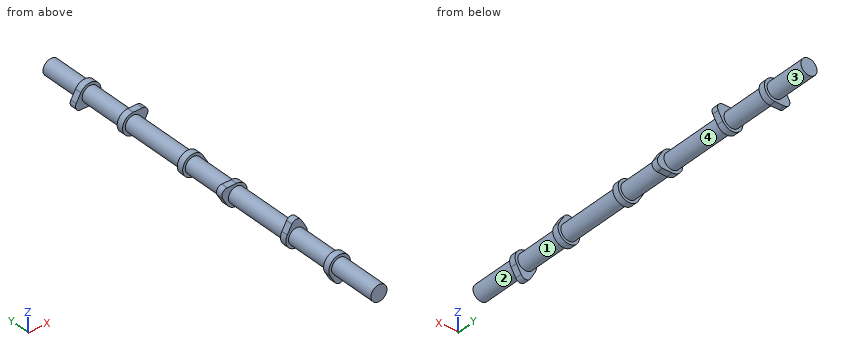
from build123d import *

# Parameters (mm, degrees)
BOSS_EXTRUDE1_DEPTH   = 3.81
LPATTERN1_COUNT       = 2
LPATTERN1_PITCH       = 60.96
BODY_MOVE_COPY1_ANGLE = 180
LPATTERN2_COUNT       = 3
LPATTERN2_PITCH       = 146.05
BODY_MOVE_COPY2_ANGLE = 120
BODY_MOVE_COPY3_ANGLE = 120
BOSS_EXTRUDE2_START   = -59.53
SKETCH5_R             = 9.5
BOSS_EXTRUDE2_DEPTH   = 464.25


with BuildPart() as part:
    # Sketch2 → Boss-Extrude1 (new, symmetric)
    with BuildSketch(Plane(origin=(0, 0, 0), x_dir=(1, 0, 0), z_dir=(0, 1, 0))):
        with BuildLine():
            Line((-5.499261314, 15.875), (-10.998522628, 6.35))
            ThreePointArc((-10.998522628, 6.35), (0, -12.7), (10.998522628, 6.35))
            Line((10.998522628, 6.35), (5.499261314, 15.875))
            ThreePointArc((5.499261314, 15.875), (0, 19.05), (-5.499261314, 15.875))
        make_face()
    extrude(amount=BOSS_EXTRUDE1_DEPTH, both=True)


with BuildPart() as lpattern1_1:
    # LPattern1: pattern copy
    add(part.part.moved(Location(Vector(0, 1, 0) * (1 * LPATTERN1_PITCH))))


with BuildPart() as lpattern1_1_1:
    # Body-Move_Copy1: moved
    add(lpattern1_1.part.rotate(Axis((0, 0, 0), (0, 1, 0)), BODY_MOVE_COPY1_ANGLE))


with BuildPart() as lpattern2_1:
    # LPattern2: pattern copy
    add(part.part.moved(Location(Vector(0, 1, 0) * (1 * LPATTERN2_PITCH))))


with BuildPart() as lpattern2_2:
    # LPattern2: pattern copy
    add(part.part.moved(Location(Vector(0, 1, 0) * (2 * LPATTERN2_PITCH))))


with BuildPart() as lpattern2_3:
    # LPattern2: pattern copy
    add(lpattern1_1_1.part.moved(Location(Vector(0, 1, 0) * (1 * LPATTERN2_PITCH))))


with BuildPart() as lpattern2_4:
    # LPattern2: pattern copy
    add(lpattern1_1_1.part.moved(Location(Vector(0, 1, 0) * (2 * LPATTERN2_PITCH))))


with BuildPart() as lpattern2_1_1:
    # Body-Move_Copy2: moved
    add(lpattern2_1.part.rotate(Axis((0, 0, 0), (0, 1, 0)), BODY_MOVE_COPY2_ANGLE))


with BuildPart() as lpattern2_3_1:
    # Body-Move_Copy2: moved
    add(lpattern2_3.part.rotate(Axis((0, 0, 0), (0, 1, 0)), BODY_MOVE_COPY2_ANGLE))


with BuildPart() as lpattern2_4_1:
    # Body-Move_Copy3: moved
    add(lpattern2_4.part.rotate(Axis((0, 0, 0), (0, -1, 0)), BODY_MOVE_COPY3_ANGLE))


with BuildPart() as lpattern2_2_1:
    # Body-Move_Copy3: moved
    add(lpattern2_2.part.rotate(Axis((0, 0, 0), (0, -1, 0)), BODY_MOVE_COPY3_ANGLE))


with BuildPart() as part_1:
    add(part.part)

    add(lpattern1_1_1.part)  # Boss-Extrude2 merges LPattern1_1

    add(lpattern2_1_1.part)  # Boss-Extrude2 merges LPattern2_1

    add(lpattern2_2_1.part)  # Boss-Extrude2 merges LPattern2_2

    add(lpattern2_3_1.part)  # Boss-Extrude2 merges LPattern2_3

    add(lpattern2_4_1.part)  # Boss-Extrude2 merges LPattern2_4
    # Sketch5 → Boss-Extrude2 (add)
    with BuildSketch(Plane(origin=(0, 0, 0), x_dir=(1, 0, 0), z_dir=(0, 1, 0)).offset(BOSS_EXTRUDE2_START)):
        with Locations(Location((0, 0, 0), (0, 0, 270))):
            Circle(SKETCH5_R)
    extrude(amount=BOSS_EXTRUDE2_DEPTH)


solid = part_1.part
Geometry: final body of the model. Coordinates: model frame, mm. Face numbers are marked on the shaded views. A direction names the side the tool comes from. Coordinates: 2 decimals unless noted, no trailing zeros. Order: outer loops, then holes, each group sorted by start corner. A loop starts at its lowest first (then second) coordinate and runs counter-clockwise, first axis right, second up.
(1) First-contact query: pin 1 (4 mm diameter, centred on x = 11, z = 12.5, fed in from +Y); pin 2 (1 mm diameter, centred on x = -2.5, y = 197, fed in from -Z); pin 3 (8.5 mm diameter, centred on x = -6.5, y = 145, fed in from +Z). Flat tips, straight axial feed; report the tip coordinate or a pass-through.
(2) Material intervals for probe 1 along Y at (x, z) = (8, 7.5); probe 2 along Y at (x, z) = (14, -0.5); probe 3 along X at (y, z) = (296, -7), sorted ascending.
(3) Draft query along Y for the marked faces 1 and 2. Return one class per face: pulls with the +Y half, pulls with the -Y half, needs draft (parallel to the pull), parting line crosses it, or undercut.
(4) Section query A-A (y = 231). Return the cut outline in (x, z), plus the area to 3 significant figures.
(5) Access query for the marked faces 3 and 4. Directions: +Z, -Z, +X, -X, +Y, -Y. A direction counts if a zero-diameter tool reaches every point of the face in a straight line with its end or side. Return the directions, or none.
Solution:
1. pin 1: stops at y = 295.91
1. pin 2: stops at z = -9.29
1. pin 3: stops at z = 12.7
2. probe 1: y = -3.81 to 3.81, 57.15 to 64.77, 142.24 to 149.86, 203.2 to 210.82, 288.29 to 295.91, 349.25 to 356.87
2. probe 2: y = 203.2 to 210.82, 288.29 to 295.91
2. probe 3: x = -6.42 to 6.42
3. face 1: undercut
3. face 2: needs draft
4. outline: circle Ø19 at (0, 0)
4. area: 284 mm2
5. face 3: +Y
5. face 4: none
